from build123d import *

# Parameters (mm, degrees)
SKETCH_1_R          = 1.05
SKETCH_1_W          = 12.2
SKETCH_1_H          = 22.2
EXTRUDE_1_DEPTH     = 5.5
CUT_EXTRUDE_1_DEPTH = 32.778294479
FILLET_1_R          = 10


with BuildPart() as part:
    # ｽｹｯﾁ1 → ﾎﾞｽ - 押し出し1 (new body)
    with BuildSketch(Plane.XY):
        Polygon((-10, -18.9), (3, -18.9), (7, -26.9), (16, -26.9), (16, 26.1), (-10, 26.1), align=None)
        with Locations((0, -13.75)):
            Circle(SKETCH_1_R, mode=Mode.SUBTRACT)
        with Locations((0, 13.75)):
            Circle(SKETCH_1_R, mode=Mode.SUBTRACT)
        with Locations((11, -17.45)):
            Circle(SKETCH_1_R, mode=Mode.SUBTRACT)
        with Locations((11, -11.45)):
            Circle(SKETCH_1_R, mode=Mode.SUBTRACT)
        Rectangle(SKETCH_1_W, SKETCH_1_H, mode=Mode.SUBTRACT)
    extrude(amount=EXTRUDE_1_DEPTH)

    # ｽｹｯﾁ2 → ｶｯﾄ - 押し出し1 (cut, through all)
    with BuildSketch(Plane.XY.offset(5.5)):
        with BuildLine():
            Line((-10, 20.371887242), (-10, 26.1))
            Line((-10, 26.1), (16, 26.1))
            Line((16, 26.1), (16, 24.844230428))
            ThreePointArc((16, 24.844230428), (2.693348244, 24.390781073), (-10, 20.371887242))
        make_face()
    extrude(amount=-CUT_EXTRUDE_1_DEPTH, mode=Mode.SUBTRACT)

    # ﾌｨﾚｯﾄ1
    fillet_1_edges = [part.edges().sort_by_distance(p)[0] for p in [
        (-10, -18.9, 2.75),
    ]]
    fillet(fillet_1_edges, radius=FILLET_1_R)


solid = part.part
Build history of the part. All positions in model axes, mm. A direction names the side the tool comes from. Give positions to 0.01 mm unless a question says otherwise; leave off trailing zeros. Order: outer loops, then holes, each group sorted by start corner. A loop starts at its lowest first (then second) coordinate and runs counter-clockwise, first axis right, second up. Notation, with made-up numbers: M 22.25,24 L 27.25,24 A27 ccw 27.25,52 Z; hole C 49.25,-22 d2. An arc over 180 degrees is marked long. Use one line per item in the form item = value.
1) Saw through at C-C (z = 4.8). Give the cut face in (x, y).
Calculated:
outline = M -10,-8.9 A10 ccw 0,-18.9 L 3,-18.9 L 7,-26.9 L 16,-26.9 L 16,24.84 A49 ccw -10,20.37 Z; hole M -6.1,-11.1 L 6.1,-11.1 L 6.1,11.1 L -6.1,11.1 Z; hole C 0,-13.75 d2.1; hole C 0,13.75 d2.1; hole C 11,-17.45 d2.1; hole C 11,-11.45 d2.1
2) Drop flat-ended pins along their axis: pin 1 (3 mm diameter, centred on x = -2, z = 4, fed in from -Y); pin 2 (1 mm diameter, centred on x = -1.5, z = 1, fed in from +Y); pin 3 (1 mm diameter, centred on x = 3.5, z = 3, fed in from +Y). Give the stop position or say it passes through.
Calculated:
pin_1 = -18.89
pin_2 = 23.61
pin_3 = 24.6
3) Saw through at B-B (y = -5). Give the cut face in (x, z).
Calculated:
outline = M -10,0 L -6.1,0 L -6.1,5.5 L -10,5.5 Z; M 6.1,0 L 16,0 L 16,5.5 L 6.1,5.5 Z
4) Saw through at A-A (x = 11). Give the cut face in (y, z).
Calculated:
outline = M -26.9,0 L -18.5,0 L -18.5,5.5 L -26.9,5.5 Z; M -16.4,0 L -12.5,0 L -12.5,5.5 L -16.4,5.5 Z; M -10.4,0 L 25.1,0 L 25.1,5.5 L -10.4,5.5 Z
5) Probe probe 1 along Y at (x, z) = (0, 2.8); probe 2 along Y at (x, z) = (11, 5.05); probe 3 along X at (y, z) = (-5, 2.15). List the from-to ranges inside material, lowest first.
Calculated:
probe_1 = -18.9 to -14.8, -12.7 to -11.1, 11.1 to 12.7, 14.8 to 23.85
probe_2 = -26.9 to -18.5, -16.4 to -12.5, -10.4 to 25.1
probe_3 = -10 to -6.1, 6.1 to 16
6) Two-plate mould, pull along Y, no slides. Class faces 4 (the face through (9, -1, 0)), 5 (the face through (2.878, 24.422, 2.788)), 6 (the face through (12, -11.13, 2.71)): released by +Y, released by -Y, zero draft, split by the parting line, or undercut.
Calculated:
face_4 = zero draft
face_5 = released by +Y
face_6 = undercut
7) Saw through at D-D (x = 5). Give the cut face in (y, z), plus the area to 3 significant figures.
Calculated:
outline = M -22.9,0 L -11.1,0 L -11.1,5.5 L -22.9,5.5 Z; M 11.1,0 L 24.73,0 L 24.73,5.5 L 11.1,5.5 Z
area = 140 mm2
8) Tool access for faces 1 (the face through (1, -18.9, 3)), 2 (the face through (16, -1, 3)), 3 (the face through (0, 11.1, 3)): list every direction of +Z, -Z, +X, -X, +Y, -Y with a clear straight run to the whole face (end or side of a thin tool).
Calculated:
face_1 = +Z, -Z, -X, -Y
face_2 = +Z, -Z, +X, +Y, -Y
face_3 = +Z, -Z
